```python
from build123d import *


# Not quite as in the source:
# - a pattern or mirror of a feature is missing from the dataset's text; its kind, count and spacing are read off the source's solid


with BuildPart() as f1:
    # F0 (on Front) → F1 (revolve)
    with BuildSketch(Plane.XZ):
        with BuildLine():
            ThreePointArc((0, 25), (2.5, 24.3301270189), (4.3301270189, 22.5))
            Line((4.3301270189, 22.5), (17.3205080757, 0))
            Line((17.3205080757, 0), (20, 0))
            Line((20, 0), (20, 10))
            ThreePointArc((20, 10), (14.1421356237, 24.1421356237), (0, 30))
            Line((0, 30), (0, 25))
        make_face()
    revolve(axis=Axis((0, 0, 15), (0, 0, 1)))

    # F2 (on Front) → F3 (revolve)
    with BuildSketch(Plane.XZ):
        with BuildLine():
            Line((15.1763809021, 46.6390246015), (9.3060056246, 24.7304858066))
            Line((9.3060056246, 24.7304858066), (13.1697089298, 23.6952096262))
            Line((13.1697089298, 23.6952096262), (17.8826102498, 41.2839968035))
            ThreePointArc((17.8826102498, 41.2839968035), (21.1445422637, 47.2563170454), (16.7292951727, 52.4345795592))
            Line((16.7292951727, 52.4345795592), (15.1763809021, 46.6390246015))
        make_face()
    f3 = revolve(axis=Axis((12.2411932633, 0, 35.684755204), (-0.2588190451, 0, -0.9659258263)))

    # F3_copies: F3 across plane
    add(f3.mirror(Plane(origin=(-2.2e-05, 0, 0), x_dir=(0, 0, -1), z_dir=(-1, 0, 0))))


solid = f1.part
```
The model under review builds one solid part; all positions refer to its coordinate system, in mm. Round coordinates to 2 decimals unless told otherwise and drop trailing zeros. Order: outer loops, then holes, each group sorted by start corner. A loop starts at its lowest first (then second) coordinate and runs counter-clockwise, first axis right, second up.
Item 1: Add section C-C, the plane z = 19. State the section outline as (x, y) points.
Working result:
outline: circle Ø35.72 at (0, 0); hole circle Ø12.7 at (0, 0)
Item 2: To check wall thickness, follow probe 1 along X at (y, z) = (-5.5, 15); probe 2 along X at (y, z) = (-5.5, 7); probe 3 along Z at (x, y) = (9, 7.5). State the ranges of each line that lie inside material, in increasing order.
Working result:
probe 1: x = -18.57 to -6.69, 6.69 to 18.57
probe 2: x = -19.23 to -12.09, 12.09 to 19.23
probe 3: z = 9.71 to 26.21
Item 3: Add section B-B, the plane y = 0. State the section outline as (x, z) points, and give its area (3 significant figures).
Working result:
outline: (-20, 0) - (-17.32, 0) - (-4.33, 22.5) arc R5 cw to (4.33, 22.5) - (17.32, 0) - (20, 0) - (20, 10) arc R20 ccw to (13.46, 24.79) - (17.88, 41.28) arc R6 ccw (long way) to (10.16, 43.35) - (6.3, 28.98) arc R20 ccw to (-6.3, 28.98) - (-10.16, 43.35) arc R6 ccw (long way) to (-17.88, 41.28) - (-13.46, 24.79) arc R20 ccw to (-20, 10) - close
area: 986 mm2
Item 4: Add section A-A, the plane x = 0. State the section outline as (y, z) points.
Working result:
outline: (-20, 0) - (-17.32, 0) - (-4.33, 22.5) arc R5 cw to (4.33, 22.5) - (17.32, 0) - (20, 0) - (20, 10) arc R20 ccw to (-20, 10) - close
Item 5: Draft analysis for pull direction X (two halves, no side actions). For faces 1 (the conical face through (-1.74, -7.84, 16.09)), 2 (the cylindrical face through (-4.336, -19.524, 5.07)), 3 (the flat face through (15, 9, 0)), state which applies: released by +X, released by -X, zero draft, split by the parting line, or undercut.
Working result:
face 1: undercut
face 2: split by the parting line
face 3: zero draft
Item 6: For pin 1 (3 mm diameter, centred on y = 6, z = 10, fed in from +X); pin 2 (2 mm diameter, centred on y = -11, z = 22, fed in from +X); pin 3 (1 mm diameter, centred on y = 0.5, z = 8, fed in from +X), all flat-tipped, find the tip position at first contact; note any pin that passes through.
Working result:
pin 1: stops at x = 19.49
pin 2: stops at x = 12.91
pin 3: stops at x = 20
